Work out the finished part from the listing and answer in its coordinate system (mm). Face numbers are marked on the shaded views. A direction names the side the tool comes from. Round coordinates to 2 decimals unless told otherwise and drop trailing zeros. Write each loop counter-clockwise with the first axis right and the second up, starting at its lowest first coordinate (ties: lowest second). Pieces come first, ordered by that corner, then holes. Notation, with made-up numbers: (-39, 49) - (0, 49) arc R5 cw to (0, 53) - close; hole circle Ø8 at (62.5, 71.25). An arc over 180 degrees is marked (long way). Answer as a JSON object with one key per item and string values.
```python
from build123d import *

# Parameters (mm, degrees)
SKETCH1_W                      = 60
SKETCH1_H                      = 42
BOSS_EXTRUDE1_DEPTH            = 12
CUT_EXTRUDE2_REACH             = 14
SKETCH3_R                      = 11.5
SKETCH3_R_2                    = 4
CUT_EXTRUDE2_DIRECTION_2_DEPTH = 1
CHAMFER1_SIZE                  = 13
CUT_EXTRUDE4_REACH             = 14
SKETCH5_W                      = 7
SKETCH5_H                      = 4
CUT_EXTRUDE4_DIRECTION_2_DEPTH = 1
SKETCH4_R                      = 2.25
CUT_EXTRUDE3_DEPTH             = 7.5


with BuildPart() as part:
    # Sketch1 → Boss-Extrude1 (new body)
    with BuildSketch(Plane(origin=(0, 0, 0), x_dir=(1, 0, 0), z_dir=(0, 1, 0))):
        Rectangle(SKETCH1_W, SKETCH1_H)
    extrude(amount=BOSS_EXTRUDE1_DEPTH)

    # Sketch3 → Cut-Extrude2 (cut, up to next)
    with BuildSketch(Plane(origin=(0, 12, 0), x_dir=(1, 0, 0), z_dir=(0, 1, 0)), mode=Mode.PRIVATE) as cut_extrude2_sk1:
        Circle(SKETCH3_R)
    cut_extrude2_tool1 = extrude(cut_extrude2_sk1.sketch, amount=-CUT_EXTRUDE2_REACH, mode=Mode.PRIVATE) & part.part
    add(cut_extrude2_tool1.solids().sort_by_distance((0, 12, 0))[0], mode=Mode.SUBTRACT)
    # Sketch3 → Cut-Extrude2 (cut, up to next)
    with BuildSketch(Plane(origin=(0, 12, 0), x_dir=(1, 0, 0), z_dir=(0, 1, 0)), mode=Mode.PRIVATE) as cut_extrude2_sk2:
        with Locations((20.75, 0)):
            Circle(SKETCH3_R_2)
    cut_extrude2_tool2 = extrude(cut_extrude2_sk2.sketch, amount=-CUT_EXTRUDE2_REACH, mode=Mode.PRIVATE) & part.part
    add(cut_extrude2_tool2.solids().sort_by_distance((20.75, 12, 0))[0], mode=Mode.SUBTRACT)
    # Sketch3 → Cut-Extrude2 (cut, up to next)
    with BuildSketch(Plane(origin=(0, 12, 0), x_dir=(1, 0, 0), z_dir=(0, 1, 0)), mode=Mode.PRIVATE) as cut_extrude2_sk3:
        with Locations((-20.75, 0)):
            Circle(SKETCH3_R_2)
    cut_extrude2_tool3 = extrude(cut_extrude2_sk3.sketch, amount=-CUT_EXTRUDE2_REACH, mode=Mode.PRIVATE) & part.part
    add(cut_extrude2_tool3.solids().sort_by_distance((-20.75, 12, 0))[0], mode=Mode.SUBTRACT)

    # Sketch3 → Cut-Extrude2 direction 2 (cut)
    with BuildSketch(Plane(origin=(0, 12, 0), x_dir=(1, 0, 0), z_dir=(0, 1, 0))):
        Circle(SKETCH3_R)
        with Locations((20.75, 0)):
            Circle(SKETCH3_R_2)
        with Locations((-20.75, 0)):
            Circle(SKETCH3_R_2)
    extrude(amount=CUT_EXTRUDE2_DIRECTION_2_DEPTH, mode=Mode.SUBTRACT)

    # Chamfer1
    chamfer1_edges = [part.edges().sort_by_distance(p)[0] for p in [
        (30, 6, 21),
        (-30, 6, 21),
    ]]
    chamfer(chamfer1_edges, length=CHAMFER1_SIZE)

    # Sketch5 → Cut-Extrude4 (cut, up to next)
    with BuildSketch(Plane(origin=(0, 12, 0), x_dir=(1, 0, 0), z_dir=(0, 1, 0)), mode=Mode.PRIVATE) as cut_extrude4_sk1:
        with Locations((24, 15)):
            Rectangle(SKETCH5_W, SKETCH5_H)
    cut_extrude4_tool1 = extrude(cut_extrude4_sk1.sketch, amount=-CUT_EXTRUDE4_REACH, mode=Mode.PRIVATE) & part.part
    add(cut_extrude4_tool1.solids().sort_by_distance((24, 12, -15))[0], mode=Mode.SUBTRACT)
    # Sketch5 → Cut-Extrude4 (cut, up to next)
    with BuildSketch(Plane(origin=(0, 12, 0), x_dir=(1, 0, 0), z_dir=(0, 1, 0)), mode=Mode.PRIVATE) as cut_extrude4_sk2:
        with Locations((6, 15)):
            Rectangle(SKETCH5_W, SKETCH5_H)
    cut_extrude4_tool2 = extrude(cut_extrude4_sk2.sketch, amount=-CUT_EXTRUDE4_REACH, mode=Mode.PRIVATE) & part.part
    add(cut_extrude4_tool2.solids().sort_by_distance((6, 12, -15))[0], mode=Mode.SUBTRACT)
    # Sketch5 → Cut-Extrude4 (cut, up to next)
    with BuildSketch(Plane(origin=(0, 12, 0), x_dir=(1, 0, 0), z_dir=(0, 1, 0)), mode=Mode.PRIVATE) as cut_extrude4_sk3:
        with Locations((-6, 15)):
            Rectangle(SKETCH5_W, SKETCH5_H)
    cut_extrude4_tool3 = extrude(cut_extrude4_sk3.sketch, amount=-CUT_EXTRUDE4_REACH, mode=Mode.PRIVATE) & part.part
    add(cut_extrude4_tool3.solids().sort_by_distance((-6, 12, -15))[0], mode=Mode.SUBTRACT)
    # Sketch5 → Cut-Extrude4 (cut, up to next)
    with BuildSketch(Plane(origin=(0, 12, 0), x_dir=(1, 0, 0), z_dir=(0, 1, 0)), mode=Mode.PRIVATE) as cut_extrude4_sk4:
        with Locations((-24, 15)):
            Rectangle(SKETCH5_W, SKETCH5_H)
    cut_extrude4_tool4 = extrude(cut_extrude4_sk4.sketch, amount=-CUT_EXTRUDE4_REACH, mode=Mode.PRIVATE) & part.part
    add(cut_extrude4_tool4.solids().sort_by_distance((-24, 12, -15))[0], mode=Mode.SUBTRACT)

    # Sketch5 → Cut-Extrude4 direction 2 (cut)
    with BuildSketch(Plane(origin=(0, 12, 0), x_dir=(1, 0, 0), z_dir=(0, 1, 0))):
        with Locations((24, 15)):
            Rectangle(SKETCH5_W, SKETCH5_H)
        with Locations((6, 15)):
            Rectangle(SKETCH5_W, SKETCH5_H)
        with Locations((-6, 15)):
            Rectangle(SKETCH5_W, SKETCH5_H)
        with Locations((-24, 15)):
            Rectangle(SKETCH5_W, SKETCH5_H)
    extrude(amount=CUT_EXTRUDE4_DIRECTION_2_DEPTH, mode=Mode.SUBTRACT)

    # Sketch4 → Cut-Extrude3 (cut)
    with BuildSketch(Plane(origin=(0, 0, -21), x_dir=(-1, 0, 0), z_dir=(0, 0, -1))):
        with Locations((-24, 6)):
            Circle(SKETCH4_R)
        with Locations((-6, 6)):
            Circle(SKETCH4_R)
        with Locations((6, 6)):
            Circle(SKETCH4_R)
        with Locations((24, 6)):
            Circle(SKETCH4_R)
    extrude(amount=-CUT_EXTRUDE3_DEPTH, mode=Mode.SUBTRACT)


solid = part.part
```
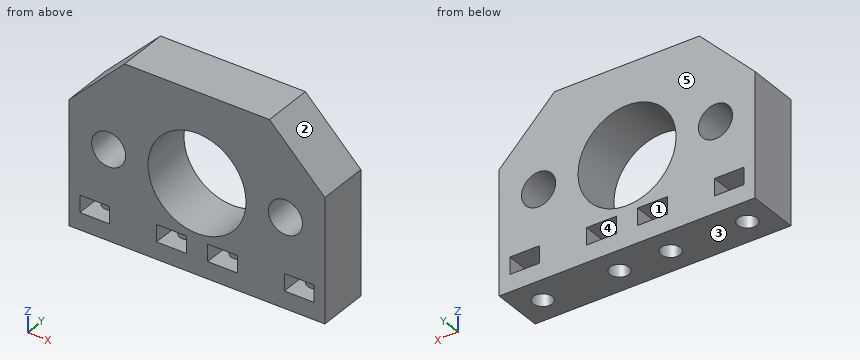
Item 1: A cutting plane is placed at C-C (z = 0). Write down the section's boundary in (x, y).
Results found:
{"outline": "(-30, 0) - (-24.75, 0) - (-24.75, 12) - (-30, 12) - close; (-16.75, 0) - (-11.5, 0) - (-11.5, 12) - (-16.75, 12) - close; (11.5, 0) - (16.75, 0) - (16.75, 12) - (11.5, 12) - close; (24.75, 0) - (30, 0) - (30, 12) - (24.75, 12) - close"}
Item 2: A cutting plane is placed at B-B (y = 1.25). Write down the section's boundary in (x, z), and give its area (3 significant figures).
Results found:
{"outline": "(-30, -21) - (30, -21) - (30, 8) - (17, 21) - (-17, 21) - (-30, 8) - close; hole (-27.5, -17) - (-20.5, -17) - (-20.5, -13) - (-27.5, -13) - close; hole circle Ø8 at (-20.75, 0); hole circle Ø23 at (0, 0); hole (-9.5, -17) - (-2.5, -17) - (-2.5, -13) - (-9.5, -13) - close; hole (2.5, -17) - (9.5, -17) - (9.5, -13) - (2.5, -13) - close; hole circle Ø8 at (20.75, 0); hole (20.5, -17) - (27.5, -17) - (27.5, -13) - (20.5, -13) - close", "area": "1,720 mm²"}
Item 3: For the marked faces 4 and 5, determine the directions among +Z, -Z, +X, -X, +Y, -Y from which every point of the face is accessible in a straight line to the end or side of a thin tool.
Results found:
{"face 4": "+Y, -Y", "face 5": "+Z, -Z, +X, -X, +Y"}
Item 4: This flat-tipped pin is pushed along its axis until it touches: P1, Ø6, axis at x = 24, y = 6, coming from the +Z side. Where does it stop, or does it pass through?
Results found:
{"P1": "z = 17"}
Item 5: Determine the mould class of the marked faces 1, 2 and 3 for opening direction Z: pulls with the +Z half, pulls with the -Z half, needs draft (parallel to the pull), parting line crosses it, or undercut.
Results found:
{"face 1": "undercut", "face 2": "pulls with the +Z half", "face 3": "pulls with the -Z half"}
Item 6: A cutting plane is placed at D-D (x = -6). Write down the section's boundary in (y, z), and give its area (3 significant figures).
Results found:
{"outline": "(0, -21) - (3.75, -21) - (3.75, -17) - (0, -17) - close; (0, -13) - (12, -13) - (12, -9.81) - (0, -9.81) - close; (0, 9.81) - (12, 9.81) - (12, 21) - (0, 21) - close; (8.25, -21) - (12, -21) - (12, -17) - (8.25, -17) - close", "area": "203 mm²"}
Item 7: A cutting plane is placed at A-A (z = -14). Write down the section's boundary in (x, y).
Results found:
{"outline": "(-30, 0) - (-27.5, 0) - (-27.5, 12) - (-30, 12) - close; (-20.5, 0) - (-9.5, 0) - (-9.5, 12) - (-20.5, 12) - close; (-2.5, 0) - (2.5, 0) - (2.5, 12) - (-2.5, 12) - close; (9.5, 0) - (20.5, 0) - (20.5, 12) - (9.5, 12) - close; (27.5, 0) - (30, 0) - (30, 12) - (27.5, 12) - close"}
Item 8: Consider line 1 along X through (y, z) = (6.5, 0); line 2 along X through (y, z) = (10.25, -6.5); line 3 along Y through (x, z) = (-24, -19.1). Determine where each line is inside the solid, lowest interval first.
Results found:
{"line 1": "-30 to -24.75, -16.75 to -11.5, 11.5 to 16.75, 24.75 to 30", "line 2": "-30 to -9.49, 9.49 to 30", "line 3": "0 to 3.75, 8.25 to 12"}
